CAD build for the part. Positions are in the model's coordinates, mm. Coordinates: 2 decimals unless noted, no trailing zeros. Order: outer loops, then holes, each group sorted by start corner. A loop starts at its lowest first (then second) coordinate and runs counter-clockwise, first axis right, second up. Notation, with made-up numbers: M 23.5,67.5 L 69.5,67.5 A26 ccw 69.5,101.5 Z; hole C -14.5,43 d11. An arc over 180 degrees is marked long. Write item = value, one per line.
from build123d import *

# Parameters (mm, degrees)
BOSS_EXTRU_1_DEPTH      = 44
ENL_V_MAT_EXTRU_1_REACH = 348
ESQUISSE2_R             = 1.75


with BuildPart() as part:
    # Esquisse1 → Boss.-Extru.1 (new body)
    with BuildSketch(Plane.XY):
        Polygon((-97.60917289, 115.219928183), (-97.60917289, 60.537847258), (174.28529528, -140.091646173), (248.39082711, -140.091646173), align=None)
    extrude(amount=BOSS_EXTRU_1_DEPTH)

    # Enlèv. mat.-Extru.1: up to this face of the body (flat: up to its plane)
    enl_v_mat_extru_1_end = Plane(part.part.faces().sort_by_distance((75.39082711, -12.435858995, 22))[0])
    # Esquisse2 → Enlèv. mat.-Extru.1 (cut, up to the picked face)
    with BuildSketch(Plane.ZY.offset(97.60917289), mode=Mode.PRIVATE) as enl_v_mat_extru_1_sk1:
        with Locations((22, 94.969928183)):
            Circle(ESQUISSE2_R)
    enl_v_mat_extru_1_tool1 = split(extrude(enl_v_mat_extru_1_sk1.sketch, amount=-ENL_V_MAT_EXTRU_1_REACH, mode=Mode.PRIVATE), bisect_by=enl_v_mat_extru_1_end, keep=Keep.BOTH, mode=Mode.PRIVATE)
    add(enl_v_mat_extru_1_tool1.solids().sort_by_distance((-97.609173, 94.969928, 22))[0], mode=Mode.SUBTRACT)


solid = part.part
(1) Slice it at A-A, the plane z = 28.5. Write the cut outline in (x, y).
Evaluation:
outline = M -97.61,60.54 L 174.29,-140.09 L 248.39,-140.09 L -97.61,115.22 Z
(2) Wall check: line 1 (Y direction, x = -75, z = 22); line 2 (X direction, y = -84, z = 30); line 3 (Y direction, x = -59, z = 5). Give the ranges that are in metal, low to high. Write a range as from..to.
Evaluation:
line_1 = 43.85..93.22, 96.72..98.54
line_2 = 98.27..172.38
line_3 = 32.05..86.73
(3) Pin check, flat tips, straight feed: pin 1 Ø1 at (y, z) = (39, 12) entering from -X; pin 2 Ø10 at (x, z) = (66.5, 9.5) entering from +Y; pin 3 Ø1.5 at (y, z) = (-67.5, 23.5) entering from -X. Stop position of each tip, or through.
Evaluation:
pin_1 = -69.1
pin_2 = -2.19
pin_3 = 74.89
(4) Slice it at B-B, the plane x = 197. Write the cut outline in (y, z), then the cut area to 3 significant figures.
Evaluation:
outline = M -140.09,0 L -102.17,0 L -102.17,44 L -140.09,44 Z
area = 1,670 mm²
